Build history of the part. All positions in model axes, mm. Face numbers are marked on the shaded views. Give positions to 0.01 mm unless a question says otherwise; leave off trailing zeros. Order: outer loops, then holes, each group sorted by start corner. A loop starts at its lowest first (then second) coordinate and runs counter-clockwise, first axis right, second up. Notation, with made-up numbers: (47, 11) - (62, 11) arc R34 ccw to (62, 42) - close; hole circle Ø10 at (13, -25.5). An arc over 180 degrees is marked (long way). Use a Markdown table: item, result.
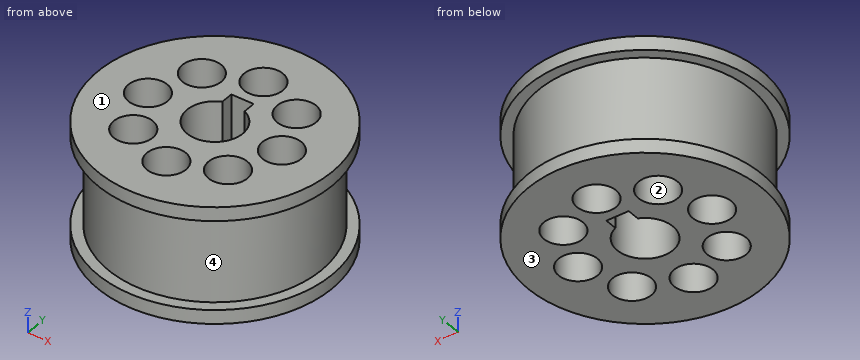
Autodesk Inventor part; units mm, degrees
ref_plane "YZ Plane" through (0, 0, 0) normal (1, 0, 0) x (0, 1, 0)
ref_plane "XZ Plane" through (0, 0, 0) normal (0, 1, 0) x (-1, 0, 0)
ref_plane "XY Plane" through (0, 0, 0) normal (0, 0, 1) x (1, 0, 0)
sketch "Sketch1" plane through (0, 0, 0) normal (0, 0, 1) x (1, 0, 0)
  circle A0 centre (0, 0) radius 21
  dimension "d0" = 42
extrude "Extrusion1" add sketch "Sketch1" along normal blind 2.5
sketch "Sketch2" plane through (0, 0, 2.5) normal (0, 0, 1) x (1, 0, 0)
  circle A0 centre (0, 0) radius 19.1
  dimension "d3" = 38.2
extrude "Extrusion2" add sketch "Sketch2" along normal blind 16
sketch "Sketch3" plane through (0, 0, 18.5) normal (0, 0, 1) x (1, 0, 0)
  circle A0 centre (0, 0) radius 21
  dimension "d6" = 42
extrude "Extrusion3" add sketch "Sketch3" along normal blind 2.5
sketch "Sketch4" plane through (0, 0, 21) normal (0, 0, 1) x (1, 0, 0)
  circle A0 centre (0, 0) radius 5
  line L0 (-2, 3.2) -> (2, 3.2)
  line L1 (2, 3.2) -> (2, 6.8)
  line L2 (2, 6.8) -> (-2, 6.8)
  line L3 (-2, 6.8) -> (-2, 3.2)
  line L4 (-2, 3.2) -> (2, 6.8) construction
  line L5 (2, 3.2) -> (-2, 6.8) construction
  point P0 (0, 5)
  dimension "d9" = 10
  dimension "d10" = 4
  dimension "d11" = 3.6
extrude "Extrusion4" cut sketch "Sketch4" against normal blind 21
sketch "Sketch5" plane through (0, 0, 21) normal (0, 0, 1) x (1, 0, 0)
  circle A0 centre (0, -12) radius 3.5
  arc A1 (-2, 4.5826) -> (2, 4.5826) centre (0, 0) ccw
  line L0 (0, 0) -> (0, -12)
  line L1 (0, 0) -> (12, 0) construction
  circle A2 centre (8.4853, -8.4853) radius 3.5
  circle A3 centre (12, 0) radius 3.5
  circle A4 centre (8.4853, 8.4853) radius 3.5
  circle A5 centre (0, 12) radius 3.5
  circle A6 centre (-8.4853, 8.4853) radius 3.5
  circle A7 centre (-12, 0) radius 3.5
  circle A8 centre (-8.4853, -8.4853) radius 3.5
  dimension "d14" = 7
  dimension "d15" = 12
  dimension "d16" = 90
  dimension "d19" = 360
extrude "Extrusion5" cut sketch "Sketch5" against normal blind 21
properties part number "24 Teeth HTD5M Pulley Steel" material "Stainless Steel"
1) Pin check, flat tips, straight feed: P1, Ø1, axis at y = 6, z = 16, coming from the +X side; P2, Ø8, axis at y = -16.5, z = 17, coming from the +X side; P3, Ø2, axis at x = 10.5, z = 5.5, coming from the +Y side; P4, Ø6, axis at x = 0, y = 0, coming from the -Z side. Stop position of each tip, or through.
Computed:
| item | result |
|---|---|
| P1 | stops at x = 18.29 |
| P2 | stops at x = 16.65 |
| P3 | stops at y = 16.57 |
| P4 | passes through |
2) Two-plate mould, pull along Z, no slides. Class the marked faces 1, 2, 3 and 4: +Z half, -Z half, draft (parallel to the pull), parting line (faces both ways), or undercut.
Computed:
| item | result |
|---|---|
| face 1 | +Z half |
| face 2 | draft |
| face 3 | -Z half |
| face 4 | undercut |
3) Wall check: line 1 (Y direction, x = 0, z = 9.75); line 2 (Y direction, x = -10, z = 18.25); line 3 (X direction, y = -3, z = 3.5). Give the ranges that are in metal, low to high. Write a range as from..to.
Computed:
| item | result |
|---|---|
| line 1 | y = -19.1..-15.5, -8.5..-5, 6.8..8.5, 15.5..19.1 |
| line 2 | y = -16.27..-11.64, -5.33..-2.87, 2.87..5.33, 11.64..16.27 |
| line 3 | x = -18.86..-13.8, -10.2..-4, 4..10.2, 13.8..18.86 |
4) Slice it at C-C (y = 7.5). Write the cut outline in (x, z), and give its area (3 significant figures).
Computed:
| item | result |
|---|---|
| outline | (-19.62, 0) - (-11.84, 0) - (-11.84, 21) - (-19.62, 21) - (-19.62, 18.5) - (-17.57, 18.5) - (-17.57, 2.5) - (-19.62, 2.5) - close; (-5.13, 0) - (5.13, 0) - (5.13, 21) - (-5.13, 21) - close; (11.84, 0) - (19.62, 0) - (19.62, 2.5) - (17.57, 2.5) - (17.57, 18.5) - (19.62, 18.5) - (19.62, 21) - (11.84, 21) - close |
| area | 476 mm² |
5) Slice it at D-D (x = 17.5). Write the cut outline in (y, z).
Computed:
| item | result |
|---|---|
| outline | (-11.61, 0) - (11.61, 0) - (11.61, 2.5) - (7.65, 2.5) - (7.65, 18.5) - (11.61, 18.5) - (11.61, 21) - (-11.61, 21) - (-11.61, 18.5) - (-7.65, 18.5) - (-7.65, 2.5) - (-11.61, 2.5) - close |
6) Slice it at B-B (y = -13.5). Write the cut outline in (x, z), and give its area (3 significant figures).
Computed:
| item | result |
|---|---|
| outline | (-16.09, 0) - (-3.16, 0) - (-3.16, 21) - (-16.09, 21) - (-16.09, 18.5) - (-13.51, 18.5) - (-13.51, 2.5) - (-16.09, 2.5) - close; (3.16, 0) - (16.09, 0) - (16.09, 2.5) - (13.51, 2.5) - (13.51, 18.5) - (16.09, 18.5) - (16.09, 21) - (3.16, 21) - close |
| area | 460 mm² |
7) Slice it at A-A (x = 0). Write the cut outline in (y, z).
Computed:
| item | result |
|---|---|
| outline | (-21, 0) - (-15.5, 0) - (-15.5, 21) - (-21, 21) - (-21, 18.5) - (-19.1, 18.5) - (-19.1, 2.5) - (-21, 2.5) - close; (-8.5, 0) - (-5, 0) - (-5, 21) - (-8.5, 21) - close; (6.8, 0) - (8.5, 0) - (8.5, 21) - (6.8, 21) - close; (15.5, 0) - (21, 0) - (21, 2.5) - (19.1, 2.5) - (19.1, 18.5) - (21, 18.5) - (21, 21) - (15.5, 21) - close |
